Work out the finished part from the listing and answer in its coordinate system (mm). Face numbers are marked on the shaded views. A direction names the side the tool comes from. Give positions to 0.01 mm unless a question says otherwise; leave off trailing zeros. Write each loop counter-clockwise with the first axis right and the second up, starting at its lowest first coordinate (ties: lowest second). Pieces come first, ordered by that corner, then holes. Notation, with made-up numbers: (-6.75, 19) - (18.25, 19) arc R29 ccw to (18.25, 55) - close; hole circle Ø1 at (-39, 2). An arc over 180 degrees is marked (long way). Write each question's results on one line, items separated by ' | '. Start each with the question number.
from build123d import *

# Parameters (mm, degrees)
F0_W      = 177.8
F0_H      = 177.8
F1_DEPTH  = 76.2
F3_DEPTH  = 156.21
F5_DEPTH  = 156.21
F6_DEPTH  = 76.9294632736
F8_DEPTH  = 21.591
F9_DEPTH  = 8.89
F2_W      = 50.8
F2_H      = 76.2
F10_DEPTH = 177.801
F4_W      = 50.8
F4_H      = 76.2
F11_DEPTH = 177.801


with BuildPart() as f1:
    # F0 (on Top) → F1 (new body)
    with BuildSketch(Plane.XY):
        Rectangle(F0_W, F0_H)
    extrude(amount=F1_DEPTH)

    # F2 (on face) → F3 (cut)
    with BuildSketch(Plane(origin=(0, 88.9, 0), x_dir=(-1, 0, 0), z_dir=(0, 1, 0))):
        Polygon((76.2, 25.4), (88.9, 25.4), (88.9, 76.2), (-11.9715367264, 76.2), (-11.9715367264, 66.5815367264), (13.4284632736, 66.5815367264), (67.31, 12.7), (76.2, 12.7), align=None)
    extrude(amount=-F3_DEPTH, mode=Mode.SUBTRACT)

    # F4 (on face) → F5 (cut)
    with BuildSketch(Plane.YZ.offset(88.9)):
        Polygon((-13.4284632736, 66.5815367264), (11.9715367264, 66.5815367264), (11.9715367264, 76.2), (-88.9, 76.2), (-88.9, 25.4), (-76.2, 25.4), (-76.2, 12.7), (-67.31, 12.7), align=None)
    extrude(amount=-F5_DEPTH, mode=Mode.SUBTRACT)

    # F6 (cut, through all): a face of the model
    f6_faces = [f1.faces().sort_by_distance(p)[0] for p in [
        (50.4357683632, 11.9715367264, 71.3907683632),
    ]]
    extrude(f6_faces, amount=-F6_DEPTH, mode=Mode.SUBTRACT)

    # F7 (on face) → F8 (cut, through all)
    with BuildSketch(Plane.YZ.offset(-67.31)):
        Polygon((-88.9, 76.2), (-88.9, 25.4), (-76.2, 25.4), (-67.31, 25.4), (-67.31, 76.2), align=None)
    extrude(amount=-F8_DEPTH, mode=Mode.SUBTRACT)

    # F9 (cut): a face of the model
    f9_faces = [f1.faces().sort_by_distance(p)[0] for p in [
        (-67.31, -71.755, 19.05),
    ]]
    extrude(f9_faces, amount=-F9_DEPTH, mode=Mode.SUBTRACT)

    # F2 (on face) → F10 (cut, through all)
    with BuildSketch(Plane(origin=(0, 88.9, 0), x_dir=(-1, 0, 0), z_dir=(0, 1, 0))):
        with Locations((-63.5, 38.1)):
            Rectangle(F2_W, F2_H)
    extrude(amount=-F10_DEPTH, mode=Mode.SUBTRACT)

    # F4 (on face) → F11 (cut, through all)
    with BuildSketch(Plane.YZ.offset(88.9)):
        with Locations((63.5, 38.1)):
            Rectangle(F4_W, F4_H)
    extrude(amount=-F11_DEPTH, mode=Mode.SUBTRACT)


solid = f1.part
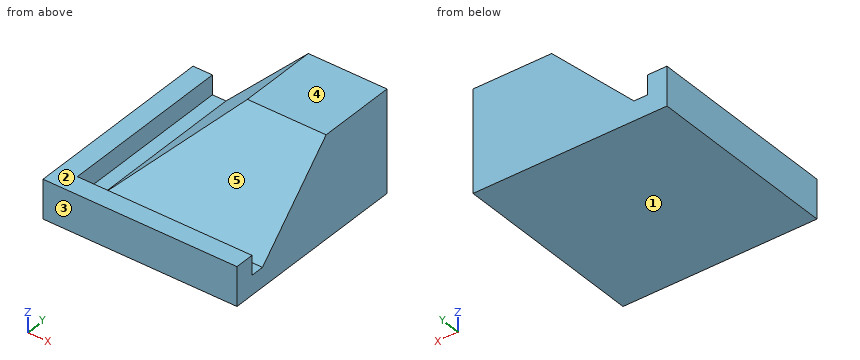
Q1. A cutting plane is placed at B-B, the plane x = -46. Write down the section's boundary in (y, z), and give its area (3 significant figures).
Q2. The mould has two halves that part along Y. Classify the marked faces 3, 4 and 5: pulls with the +Y half, pulls with the -Y half, needs draft (parallel to the pull), parting line crosses it, or undercut.
Q3. A cutting plane is placed at D-D, the plane z = 40. Write down the section's boundary in (x, y).
Q4. A cutting plane is placed at A-A, the plane z = 14.5. Write down the section's boundary in (x, y).
Q5. A tool of negligible diameter and unlimited length cuts with its end or side. For the marked faces 1 and 2, from which of +Z, -Z, +X, -X, +Y, -Y can it reach the whole face along a straight path? Write none if from no direction.
Q6. Consider L1, parallel to Z at x = 6, y = -75; L2, parallel to Z at x = 28, y = -82.5; L3, parallel to X at y = -5, z = 13.5. Determine where each line is inside the solid, lowest interval first.
Q7. Given pin 1 (4 mm diameter, centred on x = 17.5, y = -66, fed in from +Z); pin 2 (12 mm diameter, centred on x = -40.5, y = -62.5, fed in from +Z), each flat-ended and moving along its own axis, determine where each tip first touches the part or whether it passes through.
Q8. A cutting plane is placed at C-C, the plane y = -27. Write down the section's boundary in (x, z), and give its area (3 significant figures).
Result:
1) outline: (-88.9, 0) - (38.1, 0) - (38.1, 34.01) - (-46, 34.01) - (-67.31, 12.7) - (-76.2, 12.7) - (-76.2, 25.4) - (-88.9, 25.4) - close | area: 3,790 mm2
2) face 3: pulls with the -Y half | face 4: needs draft | face 5: undercut
3) outline: (-40.01, -40.01) - (38.1, -40.01) - (38.1, 38.1) - (-40.01, 38.1) - close
4) outline: (-88.9, -88.9) - (38.1, -88.9) - (38.1, -76.2) - (-76.2, -76.2) - (-76.2, 38.1) - (-88.9, 38.1) - close; (-65.51, -65.51) - (38.1, -65.51) - (38.1, 38.1) - (-65.51, 38.1) - close
5) face 1: -Z, +X, -X, +Y, -Y | face 2: +Z, -X, -Y
6) L1: z = 0 to 12.7 | L2: z = 0 to 25.4 | L3: x = -88.9 to -76.2, -66.51 to 38.1
7) pin 1: stops at z = 16.01 | pin 2: stops at z = 23.51
8) outline: (-88.9, 0) - (38.1, 0) - (38.1, 53.01) - (-27, 53.01) - (-67.31, 12.7) - (-76.2, 12.7) - (-76.2, 25.4) - (-88.9, 25.4) - close | area: 5,210 mm2
